Source: CAD feature listing. Evaluate the final solid. Frame: model axes, mm. Face numbers are marked on the shaded views. A direction names the side the tool comes from. Give positions to 0.01 mm unless a question says otherwise; leave off trailing zeros. Loops run counter-clockwise (first coordinate to the right, second up) from the corner with the lowest first, then second, coordinate; pieces in that order, holes last.
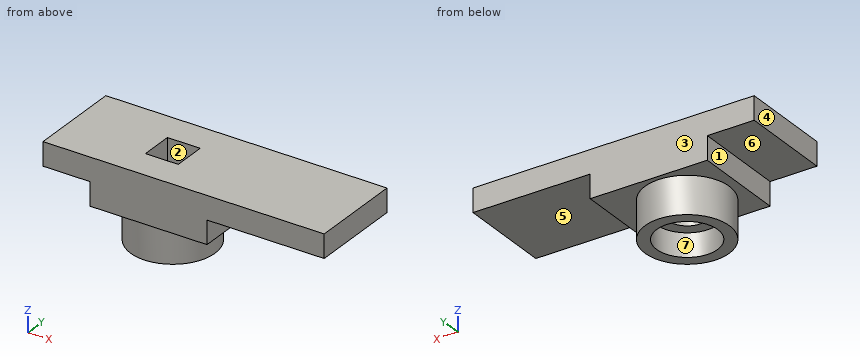
```python
from build123d import *

# Parameters (mm, degrees)
SKETCH1_W           = 60
SKETCH1_H           = 20
BOSS_EXTRUDE1_DEPTH = 10
SKETCH2_W           = 7
SKETCH2_H           = 7
CUT_EXTRUDE1_DEPTH  = 10
SKETCH3_W           = 25
SKETCH3_H           = 5
SKETCH3_W_2         = 10
CUT_EXTRUDE2_DEPTH  = 65.031242374
SKETCH5_R           = 9
BOSS_EXTRUDE2_DEPTH = 8
SKETCH6_R           = 6.51
CUT_EXTRUDE3_DEPTH  = 5
SKETCH7_R           = 4
CUT_EXTRUDE4_DEPTH  = 8


with BuildPart() as part:
    # Sketch1 → Boss-Extrude1 (new body)
    with BuildSketch(Plane.XY):
        with Locations((-30, 10)):
            Rectangle(SKETCH1_W, SKETCH1_H)
    extrude(amount=BOSS_EXTRUDE1_DEPTH)

    # Sketch2 → Cut-Extrude1 (cut)
    with BuildSketch(Plane.XY.offset(10)):
        with Locations((-39, 10)):
            Rectangle(SKETCH2_W, SKETCH2_H)
    extrude(amount=-CUT_EXTRUDE1_DEPTH, mode=Mode.SUBTRACT)

    # Sketch3 → Cut-Extrude2 (cut, through all)
    with BuildSketch(Plane(origin=(0, 0, 0), x_dir=(-1, 0, 0), z_dir=(0, -1, 0))):
        with Locations((12.5, -2.5)):
            Rectangle(SKETCH3_W, SKETCH3_H)
        with Locations((55, -2.5)):
            Rectangle(SKETCH3_W_2, SKETCH3_H)
    extrude(amount=-CUT_EXTRUDE2_DEPTH, mode=Mode.SUBTRACT)

    # Sketch5 → Boss-Extrude2 (add)
    with BuildSketch(Plane(origin=(0, 0, 0), x_dir=(-1, 0, 0), z_dir=(0, 0, -1))):
        with Locations(Location((39, 10, 0), (0, 0, 180))):
            Circle(SKETCH5_R)
    extrude(amount=BOSS_EXTRUDE2_DEPTH)

    # Sketch6 → Cut-Extrude3 (cut)
    with BuildSketch(Plane(origin=(0, 0, -8), x_dir=(-1, 0, 0), z_dir=(0, 0, -1))):
        with Locations((39, 10)):
            Circle(SKETCH6_R)
    extrude(amount=-CUT_EXTRUDE3_DEPTH, mode=Mode.SUBTRACT)

    # Sketch7 → Cut-Extrude4 (cut)
    with BuildSketch(Plane(origin=(0, 0, -3), x_dir=(-1, 0, 0), z_dir=(0, 0, -1))):
        with Locations((39, 10)):
            Circle(SKETCH7_R)
    extrude(amount=-CUT_EXTRUDE4_DEPTH, mode=Mode.SUBTRACT)


solid = part.part
```
(1) First-contact query: pin 1 (1 mm diameter, centred on y = 12, z = -4, fed in from +X); pin 2 (10.5 mm diameter, centred on x = -39, y = 10, fed in from -Z); pin 3 (3.5 mm diameter, centred on y = 10, z = 3.5, fed in from +X); pin 4 (8 mm diameter, centred on x = -55.5, y = 7, fed in from -Z). Flat tips, straight axial feed; report the tip coordinate or a pass-through.
A:
pin 1: stops at x = -30.13
pin 2: stops at z = -3
pin 3: stops at x = 0
pin 4: stops at z = 5
(2) Section A-A, the plane y = 10. Return the cut outline in (x, z).
A:
outline: (-60, 5) - (-50, 5) - (-50, 0) - (-48, 0) - (-48, -8) - (-45.51, -8) - (-45.51, -3) - (-43, -3) - (-43, 5) - (-42.5, 5) - (-42.5, 10) - (-60, 10) - close; (-35.5, 5) - (-35, 5) - (-35, -3) - (-32.49, -3) - (-32.49, -8) - (-30, -8) - (-30, 0) - (-25, 0) - (-25, 5) - (0, 5) - (0, 10) - (-35.5, 10) - close
(3) Section B-B, the plane x = -39. Return the cut outline in (y, z), then the cut area to 3 significant figures.
A:
outline: (0, 0) - (1, 0) - (1, -8) - (3.49, -8) - (3.49, -3) - (6, -3) - (6, 5) - (6.5, 5) - (6.5, 10) - (0, 10) - close; (13.5, 5) - (14, 5) - (14, -3) - (16.51, -3) - (16.51, -8) - (19, -8) - (19, 0) - (20, 0) - (20, 10) - (13.5, 10) - close
area: 180 mm2
(4) Ray query, line 1 along Y through (x, z) = (-36, 4.5); line 2 along Y through (x, z) = (-39, -7); line 3 along Z through (x, y) = (-3.5, 9.5). Return the intervals inside material, ascending.
A:
line 1: y = 0 to 6.5, 13.5 to 20
line 2: y = 1 to 3.49, 16.51 to 19
line 3: z = 5 to 10
(5) Section C-C, the plane y = 18. Return the cut outline in (x, z).
A:
outline: (-60, 5) - (-50, 5) - (-50, 0) - (-43.12, 0) - (-43.12, -8) - (-34.88, -8) - (-34.88, 0) - (-25, 0) - (-25, 5) - (0, 5) - (0, 10) - (-60, 10) - close
(6) Reachability of the marked faces 4, 5, 6 and 7 from +Z, -Z, +X, -X, +Y, -Y: full face, straight path, thin tool, end or side. Return the list, or none.
A:
face 4: +Z, -Z, -X, +Y, -Y
face 5: -Z, +X, +Y, -Y
face 6: -Z, -X, +Y, -Y
face 7: -Z
(7) Section D-D, the plane x = -19.5. Return the cut outline in (y, z).
A:
outline: (0, 5) - (20, 5) - (20, 10) - (0, 10) - close
(8) Mould query, pull axis X, two halves, no side actions, for the marked faces 1, 2 and 3. Classes: pulls with the +X half, pulls with the -X half, needs draft (parallel to the pull), parting line crosses it, or undercut.
A:
face 1: pulls with the -X half
face 2: undercut
face 3: needs draft
